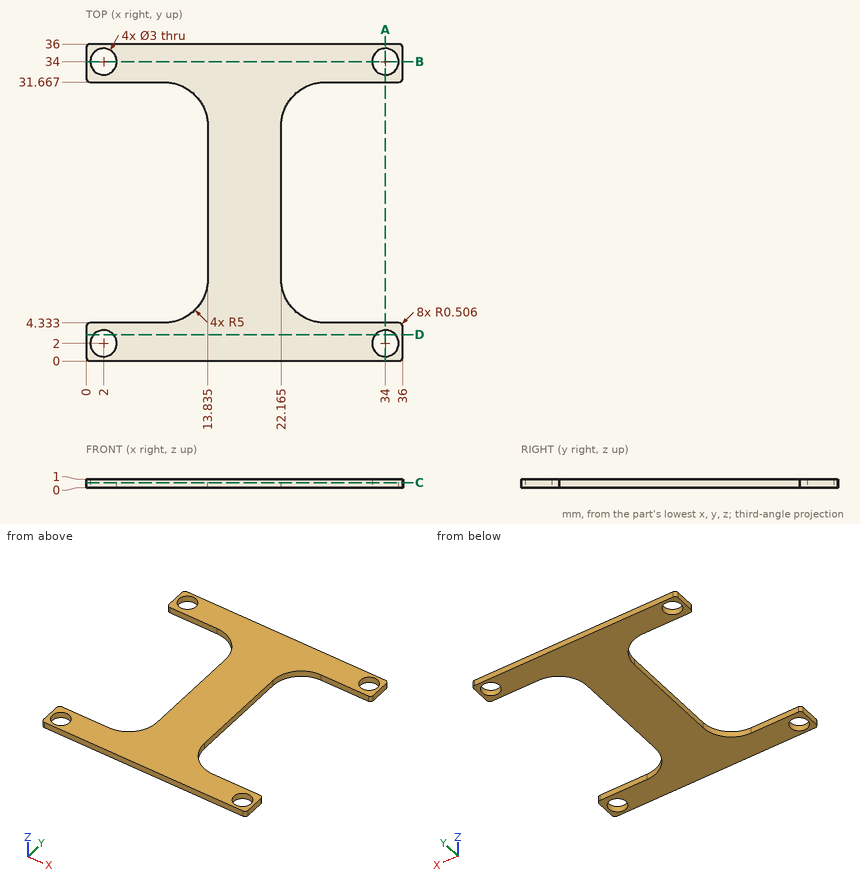
Here's the drawing with two shaded views (mm, measured from the low corner). I have some questions. Round coordinates to 2 decimals unless told otherwise and drop trailing zeros. Loops run counter-clockwise (first coordinate to the right, second up) from the corner with the lowest first, then second, coordinate; pieces in that order, holes last. Notation, with made-up numbers: (-23.75, 9.5) - (2.25, 9.5) arc R17 cw to (2.25, 40.5) - close; hole circle Ø10 at (66.5, -20.5). An arc over 180 degrees is marked (long way). Use CSV: the item, a comma, the result in double quotes. Start each with the question number.
1) If we section it at B-B on y = 34: Write out the boundary of the cut face in (x, z), plus the area to 3 significant figures.
2) If we section it at D-D on y = 3: Write out the boundary of the cut face in (x, z).
3) Please list where these lines run through material, in increasing order: probe 1 along Y at (x, z) = (34, 0.3); probe 2 along Y at (x, z) = (28, 0.8); probe 3 along Y at (x, z) = (34.5, 0.9) (1 decimal). Write a range as [from, to].
4) If we section it at C-C on z = 0.6: Write out the boundary of the cut face in (x, y) (1 decimal).
5) If we section it at A-A on x = 34: Write out the boundary of the cut face in (y, z).
Geometry results:
1,outline,"(0, 0) - (0.5, 0) - (0.5, 1) - (0, 1) - close; (3.5, 0) - (32.5, 0) - (32.5, 1) - (3.5, 1) - close; (35.5, 0) - (36, 0) - (36, 1) - (35.5, 1) - close"
1,area,"30.0 mm2"
2,outline,"(0, 0) - (0.88, 0) - (0.88, 1) - (0, 1) - close; (3.12, 0) - (32.88, 0) - (32.88, 1) - (3.12, 1) - close; (35.12, 0) - (36, 0) - (36, 1) - (35.12, 1) - close"
3,probe 1,"y = [0, 0.5], [3.5, 4.33], [31.67, 32.5], [35.5, 36]"
3,probe 2,"y = [0, 4.33], [31.67, 36]"
3,probe 3,"y = [0, 0.6], [3.4, 4.3], [31.7, 32.6], [35.4, 36]"
4,outline,"(0, 0.5) arc R0.5 ccw to (0.5, 0) - (35.5, 0) arc R0.5 ccw to (36, 0.5) - (36, 3.8) arc R0.5 ccw to (35.5, 4.3) - (27.2, 4.3) arc R5 cw to (22.2, 9.3) - (22.2, 26.7) arc R5 cw to (27.2, 31.7) - (35.5, 31.7) arc R0.5 ccw to (36, 32.2) - (36, 35.5) arc R0.5 ccw to (35.5, 36) - (0.5, 36) arc R0.5 ccw to (0, 35.5) - (0, 32.2) arc R0.5 ccw to (0.5, 31.7) - (8.8, 31.7) arc R5 cw to (13.8, 26.7) - (13.8, 9.3) arc R5 cw to (8.8, 4.3) - (0.5, 4.3) arc R0.5 ccw to (0, 3.8) - close; hole circle Ø3 at (2, 2); hole circle Ø3 at (2, 34); hole circle Ø3 at (34, 2); hole circle Ø3 at (34, 34)"
5,outline,"(0, 0) - (0.5, 0) - (0.5, 1) - (0, 1) - close; (3.5, 0) - (4.33, 0) - (4.33, 1) - (3.5, 1) - close; (31.67, 0) - (32.5, 0) - (32.5, 1) - (31.67, 1) - close; (35.5, 0) - (36, 0) - (36, 1) - (35.5, 1) - close"
